from build123d import *

# Parameters (mm, degrees)
F8_R          = 0.75
F8_R_2        = 1
F9_DEPTH      = 6.001
F9_DEPTH_BACK = 6.001
F11_SIZE      = 0.5
F12_R         = 0.5
F13_R         = 0.3


# Not quite as in the source:
# - a fillet or chamfer that OpenCascade refuses, or shapes differently, is made with other operations: its cross-section is extruded or revolved along the edge and cut away or added


with BuildPart() as f4:
    # F3 (on Front) → F4 (revolve)
    with BuildSketch(Plane.XZ):
        with BuildLine():
            Line((2.7, 6), (-2.7, 6))
            Line((-2.7, 6), (-2.7, 5.3))
            Line((-2.7, 5.3), (-4.3, 4.5))
            Line((-4.3, 4.5), (-4.3, 2.775))
            ThreePointArc((-4.3, 2.775), (-4.3878679656, 2.5628679656), (-4.6, 2.475))
            Line((-4.6, 2.475), (-16.8, 2.475))
            Line((-16.8, 2.475), (-16.8, 1.925))
            Line((-16.8, 1.925), (-27.2, 1.925))
            Line((-27.2, 1.925), (-27.2, 0))
            Line((-27.2, 0), (2.7, 0))
            Line((2.7, 0), (2.7, 6))
        make_face()
    revolve(axis=Axis((0, 0, 0), (1, 0, 0)))

    # F2 (on Front) → F5 (revolve, cut)
    with BuildSketch(Plane.XZ):
        with BuildLine():
            Line((5, 3.5), (0, 3.5))
            ThreePointArc((0, 3.5), (-2.4748737342, 2.4748737342), (-3.5, 0))
            Line((-3.5, 0), (5, 0))
            Line((5, 0), (5, 3.5))
        make_face()
    revolve(axis=Axis((0, 0, 0), (1, 0, 0)), mode=Mode.SUBTRACT)

    # F6 (on Front) → F7 (revolve, cut)
    with BuildSketch(Plane.XZ):
        Polygon((1.1386751346, 6), (-1.1386751346, 6), (-0.85, 5.5), (0.85, 5.5), align=None)
    revolve(axis=Axis((0, 0, 0), (1, 0, 0)), mode=Mode.SUBTRACT)

    # F8 (on Top) → F9 (cut, two sides)
    with BuildSketch(Plane.XY) as f9_sk:
        Circle(F8_R)
        with Locations((-14.8, 0)):
            Circle(F8_R_2)
    extrude(amount=-F9_DEPTH, mode=Mode.SUBTRACT)
    extrude(f9_sk.sketch, amount=F9_DEPTH_BACK, mode=Mode.SUBTRACT)

    # F10: chamfer of 2 x 1.4004150764 on 1 edges, made by hand

    # F10_s1 → F10_t2 (revolve, cut)
    with BuildSketch(Plane.XZ):
        Polygon((2.7, 4.9004150764), (0.7, 3.5), (2.7, 3.5), align=None)
    revolve(axis=Axis((2.7, 0, 0), (-1, 0, 0)), mode=Mode.SUBTRACT)

    # F11
    f11_edges = [f4.edges().sort_by_distance(p)[0] for p in [
        (-27.2, 0, -1.925),
    ]]
    chamfer(f11_edges, length=F11_SIZE)

    # F12
    f12_edges = [f4.edges().sort_by_distance(p)[0] for p in [
        (-4.3, 0, -4.5),
        (-2.7, 0, -5.3),
    ]]
    fillet(f12_edges, radius=F12_R)

    # F13
    f13_edges = [f4.edges().sort_by_distance(p)[0] for p in [
        (-16.8, 0, -1.925),
    ]]
    fillet(f13_edges, radius=F13_R)


solid = f4.part
The listing builds one solid part. Answer for the finished solid, in the listing's coordinates (mm). A direction names the side the tool comes from. Give positions to 0.01 mm unless a question says otherwise; leave off trailing zeros. Write each loop counter-clockwise with the first axis right and the second up, starting at its lowest first coordinate (ties: lowest second). Pieces come first, ordered by that corner, then holes. Notation, with made-up numbers: (10, 13.5) - (54, 13.5) arc R10 ccw to (54, 21.5) - close; hole circle Ø4 at (-16, 55.5). An arc over 180 degrees is marked (long way). One line per question, with ' | ' between items. Start each with the question number.
1. For faces 1 (the face through (-4.3, 3, 1)), 2 (the face through (0.01, 2.11, 5.08)), 3 (the face through (2, 0, -6)), 4 (the face through (0.3, -3.5, 0.1)), 5 (the face through (-0.75, 0.03, 4.44)), determine the directions among +Z, -Z, +X, -X, +Y, -Y from which every point of the face is accessible in a straight line to the end or side of a thin tool.
2. Straight lines are drawn through the part: line 1 (X direction, y = 0, z = 4.05); line 2 (Y direction, x = 0, z = 4); line 3 (Y direction, x = -1.25, z = 0.5). For each, find the intervals that lie inside material, in ascending order.
3. Section A-A, the plane x = -15.5 is taken. Determine the outline of the cut face in (y, z) (3 decimals).
4. Given P1, Ø2, axis at x = -8, z = 2, coming from the -Y side; P2, Ø6, axis at x = -7, y = 2, coming from the +Z side; P3, Ø2, axis at x = 0, y = 0, coming from the +Z side, each flat-ended and moving along its own axis, determine where each tip first touches the part or whether it passes through.
5. Section B-B, the plane x = -1.5 is taken. Determine the outline of the cut face in (y, z), then the cut area to 3 significant figures.
6. Section C-C, the plane x = -6.5 is taken. Determine the outline of the cut face in (y, z) (3 decimals), then the cut area to 3 significant figures.
7. Section D-D, the plane x = -21.5 is taken. Determine the outline of the cut face in (y, z) (3 decimals), then the cut area to 3 significant figures.
8. Determine the mould class of faces 6 (the face through (-27.2, 0, 0)), 7 (the face through (-2, 0, -6)), 8 (the face through (-0.75, 0.03, -4.44)) for opening direction X: +X half, -X half, draft (parallel to the pull), parting line (faces both ways), or undercut.
Result:
1) face 1: -X | face 2: none | face 3: +X, -X | face 4: +X | face 5: +Z, -Z
2) line 1: x = -4.3 to -0.75, 0.75 to 1.49 | line 2: y = -3.77 to -0.75, 0.75 to 3.77 | line 3: y = -5.98 to -3.23, 3.23 to 5.98
3) outline: (-0.714, -2.37) - (-0.714, 2.37) arc R2.475 ccw to start; (0.714, -2.37) arc R2.475 ccw to (0.714, 2.37) - close
4) P1: stops at y = -2.26 | P2: stops at z = 4.43 | P3: stops at z = 5.76
5) outline: circle Ø12 at (0, 0); hole circle Ø6.32 at (0, 0) | area: 81.7 mm2
6) outline: circle Ø4.95 at (0, 0) | area: 19.2 mm2
7) outline: circle Ø3.85 at (0, 0) | area: 11.6 mm2
8) face 6: -X half | face 7: draft | face 8: undercut
